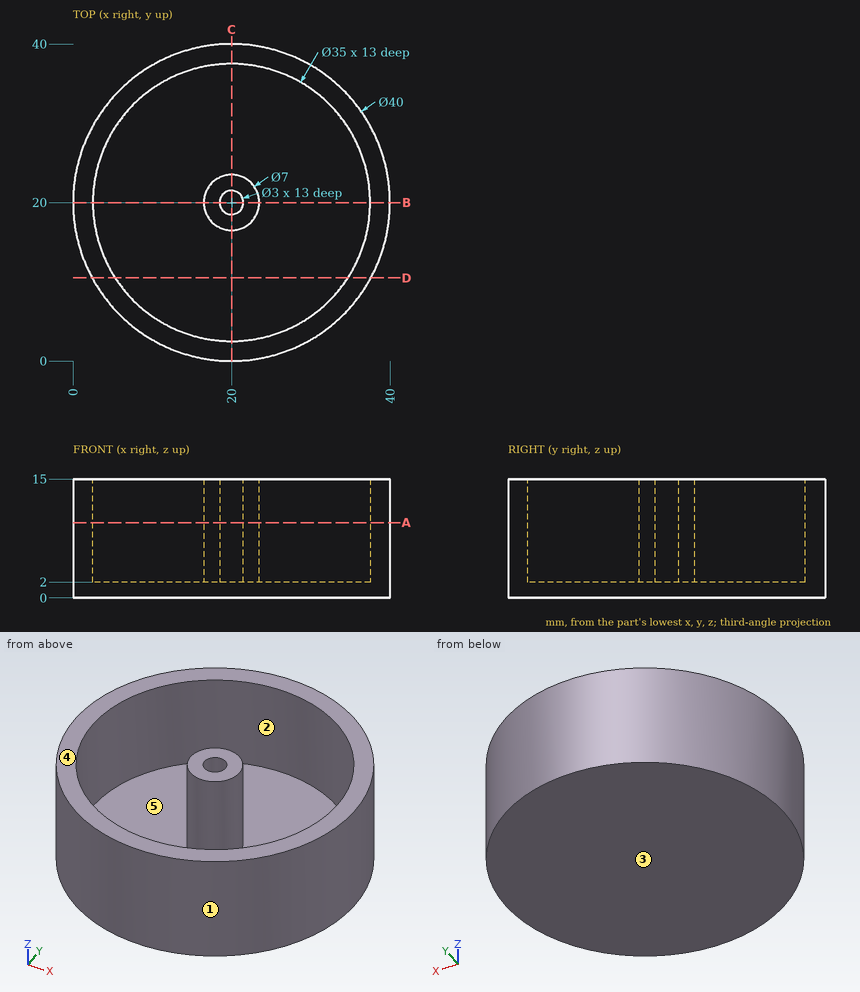
Geometry: see drawing. Coordinates: mm, zero at the bounding-box minimum. A direction names the side the tool comes from. Coordinates: 2 decimals unless noted, no trailing zeros. Loops run counter-clockwise (first coordinate to the right, second up) from the corner with the lowest first, then second, coordinate; pieces in that order, holes last. Notation, with made-up numbers: (83, 87) - (133, 87) arc R31 cw to (133, 113) - close; hole circle Ø8 at (84.5, 65.25). An arc over 180 degrees is marked (long way). Answer in a Markdown table with one row per item.
(1) Material intervals for L1, parallel to Y at x = 20, z = 9.25; L2, parallel to X at y = 18, z = 13; L3, parallel to Y at x = 20.5, z = 8.5, sorted ascending. Write a range as from..to.
Model answer:
| item | result |
|---|---|
| L1 | y = 0..2.5, 16.5..18.5, 21.5..23.5, 37.5..40 |
| L2 | x = 0.1..2.61, 17.13..22.87, 37.39..39.9 |
| L3 | y = 0.01..2.51, 16.54..18.59, 21.41..23.46, 37.49..39.99 |
(2) Pin query (flat end, axial travel): P1, Ø1, axis at x = 22, y = 27, coming from the +Z side; P2, Ø5, axis at x = 28, z = 9, coming from the -Y side; P3, Ø10.5, axis at x = 28, y = 19, coming from the +Z side; P4, Ø3, axis at x = 19, z = 13, coming from the +Y side. Return the tip coordinate at first contact, or that it passes through.
Model answer:
| item | result |
|---|---|
| P1 | stops at z = 2 |
| P2 | stops at y = 0.77 |
| P3 | stops at z = 15 |
| P4 | stops at y = 40 |
(3) Cut plane B-B on y = 20. Output: boundary loops of the cut face in (x, z), plus the area to 3 significant figures.
Model answer:
| item | result |
|---|---|
| outline | (0, 0) - (40, 0) - (40, 15) - (37.5, 15) - (37.5, 2) - (23.5, 2) - (23.5, 15) - (21.5, 15) - (21.5, 2) - (18.5, 2) - (18.5, 15) - (16.5, 15) - (16.5, 2) - (2.5, 2) - (2.5, 15) - (0, 15) - close |
| area | 197 mm² |
(4) Mould query, pull axis X, two halves, no side actions, for the marked faces 1, 2 and 3. Classes: pulls with the +X half, pulls with the -X half, needs draft (parallel to the pull), parting line crosses it, or undercut.
Model answer:
| item | result |
|---|---|
| face 1 | parting line crosses it |
| face 2 | undercut |
| face 3 | needs draft |
(5) Set-up query: the marked faces 4 and 5. Return all of +Z, -Z, +X, -X, +Y, -Y with unobstructed straight access to the full face (end or side cutting, diameter ignored); none if empty.
Model answer:
| item | result |
|---|---|
| face 4 | +Z, +X, -X, +Y, -Y |
| face 5 | +Z |
(6) Cut plane D-D on y = 10.5. Output: boundary loops of the cut face in (x, z).
Model answer:
| item | result |
|---|---|
| outline | (2.4, 0) - (37.6, 0) - (37.6, 15) - (34.7, 15) - (34.7, 2) - (5.3, 2) - (5.3, 15) - (2.4, 15) - close |
(7) Cut plane A-A on z = 9.5. Output: boundary loops of the cut face in (x, y).
Model answer:
| item | result |
|---|---|
| outline | circle Ø40 at (20, 20); circle Ø7 at (20, 20); hole circle Ø35 at (20, 20); hole circle Ø3 at (20, 20) |
